from build123d import *

# Parameters (mm, degrees)
F1_DEPTH = 13
F2_W     = 110
F2_H     = 20
F3_DEPTH = 25
F4_W     = 150
F4_H     = 25
F5_DEPTH = 15
F6_R     = 7.5
F7_DEPTH = 25


with BuildPart() as f1:
    # F0 (on Front) → F1 (new body)
    with BuildSketch(Plane.XZ):
        with BuildLine():
            Line((133.362575, 102.236308), (-123.637425, 102.236308))
            ThreePointArc((-123.637425, 102.236308), (-137.779561, 96.378444), (-143.637425, 82.236308))
            Line((-143.637425, 82.236308), (-143.637425, -61.831403))
            Line((-143.637425, -61.831403), (-143.637425, -81.831403))
            Line((-143.637425, -81.831403), (-143.637425, -87.763692))
            ThreePointArc((-143.637425, -87.763692), (-137.779561, -101.905827), (-123.637425, -107.763692))
            Line((-123.637425, -107.763692), (133.362575, -107.763692))
            ThreePointArc((133.362575, -107.763692), (147.50471, -101.905827), (153.362575, -87.763692))
            Line((153.362575, -87.763692), (153.362575, -81.831403))
            Line((153.362575, -81.831403), (153.362575, -61.831403))
            Line((153.362575, -61.831403), (153.362575, 82.236308))
            ThreePointArc((153.362575, 82.236308), (147.50471, 96.378444), (133.362575, 102.236308))
        make_face()
    extrude(amount=F1_DEPTH)

    # F2 (on face) → F3 (cut)
    with BuildSketch(Plane.XZ.offset(13)):
        with Locations((-88.637425, -65.322807)):
            Rectangle(F2_W, F2_H)
        with Locations((98.362575, -65.322807)):
            Rectangle(F2_W, F2_H)
    extrude(amount=-F3_DEPTH, mode=Mode.SUBTRACT)

    # F4 (on face) → F5 (join)
    with BuildSketch(Plane.XZ.offset(13)):
        with Locations((-68.637425, 12.5)):
            Rectangle(F4_W, F4_H)
    extrude(amount=F5_DEPTH)

    # F6 (on face) → F7 (join)
    with BuildSketch(Plane.XZ.offset(13)):
        with Locations((-111.137425, 82.236308)):
            Circle(F6_R)
        with Locations((-91.274098, 82.236308)):
            Circle(F6_R)
        with Locations((-55.741716, 82.236308)):
            Circle(F6_R)
        with Locations((-35.15286, 82.236308)):
            Circle(F6_R)
        with Locations((-4.601658, 82.236308)):
            Circle(F6_R)
        with Locations((22.960842, 82.236308)):
            Circle(F6_R)
    extrude(amount=F7_DEPTH)


solid = f1.part
Could you check a few things on this model? Use its own coordinates, in mm. A direction names the side the tool comes from. Coordinates: 2 decimals unless noted, no trailing zeros. Write each loop counter-clockwise with the first axis right and the second up, starting at its lowest first coordinate (ties: lowest second). Pieces come first, ordered by that corner, then holes. Notation, with made-up numbers: (6, 62) - (47, 62) arc R35 cw to (47, 100) - close; hole circle Ø8 at (-28, 42.25). An arc over 180 degrees is marked (long way). Write item = value, one per line.
1) For faces 1 (the flat face through (43.363, -7, -65)), 2 (the cylindrical face through (-103.984, -25.325, 84.489)), 3 (the flat face through (6.363, -20, 12)), 4 (the flat face through (-33.637, -7, -65)), 5 (the flat face through (-70, -20, 25)), which set-ups out of +Z, -Z, +X, -X, +Y, -Y let a thin tool reach every point of the face, with its end or its side?
Result set:
face_1 = +X, +Y, -Y
face_2 = -Y
face_3 = +Z, -Z, +X, -Y
face_4 = -X, +Y, -Y
face_5 = +X, -X, -Y
2) Please list where these lines run through material, in increasing order: line 1 (Z direction, x = 67, y = -12); line 2 (Y direction, x = 95, z = 18); line 3 (X direction, y = -2.5, z = -68). Write a range as [from, to].
Result set:
line_1 = [-107.76, -75.32], [-55.32, 102.24]
line_2 = [-13, 0]
line_3 = [-33.64, 43.36]
3) Suppose I cut it at B-B on x = -90. Please give me the cut outline in (y, z), plus the area to 3 significant figures.
Result set:
outline = (-38, 74.85) - (-13, 74.85) - (-13, 25) - (-28, 25) - (-28, 0) - (-13, 0) - (-13, -55.32) - (0, -55.32) - (0, 102.24) - (-13, 102.24) - (-13, 89.63) - (-38, 89.63) - close; (-13, -107.76) - (0, -107.76) - (0, -75.32) - (-13, -75.32) - close
area = 3,210 mm2
4) We'd pull the mould along Z, two halves only. Please class faces 6 (the flat face through (-70, -28, 13)), 7 (the flat face through (98, -7, -55.323)), 8 (the flat face through (-89, -7, -75.323)), 9 (the flat face through (-70, -20, 0)): +Z half, -Z half, draft (parallel to the pull), parting line (faces both ways), or undercut.
Result set:
face_6 = draft
face_7 = undercut
face_8 = undercut
face_9 = -Z half
5) Will these pins go through, and if not, where does the flat tip stop? pin 1 Ø7.5 at (x, y) = (-85.5, -23) entering from +Z; pin 2 Ø4 at (x, z) = (45.5, 52.5) entering from -Y; pin 3 Ø7.5 at (x, y) = (-69, -21.5) entering from -Z.
Result set:
pin_1 = 89.46
pin_2 = -13
pin_3 = 0
6) Suppose I cut it at C-C on y = -9.5. Please give me the cut outline in (x, z).
Result set:
outline = (-143.64, -87.76) arc R20 ccw to (-123.64, -107.76) - (133.36, -107.76) arc R20 ccw to (153.36, -87.76) - (153.36, -75.32) - (43.36, -75.32) - (43.36, -55.32) - (153.36, -55.32) - (153.36, 82.24) arc R20 ccw to (133.36, 102.24) - (-123.64, 102.24) arc R20 ccw to (-143.64, 82.24) - (-143.64, -55.32) - (-33.64, -55.32) - (-33.64, -75.32) - (-143.64, -75.32) - close
7) Suppose I cut it at D-D on x = 123. Please give me the cut outline in (y, z).
Result set:
outline = (-13, -107.76) - (0, -107.76) - (0, -75.32) - (-13, -75.32) - close; (-13, -55.32) - (0, -55.32) - (0, 102.24) - (-13, 102.24) - close
8) Suppose I cut it at A-A on y = -23. Please give me the cut outline in (x, z).
Result set:
outline = (-143.64, 0) - (6.36, 0) - (6.36, 25) - (-143.64, 25) - close; circle Ø15 at (-111.14, 82.24); circle Ø15 at (-91.27, 82.24); circle Ø15 at (-55.74, 82.24); circle Ø15 at (-35.15, 82.24); circle Ø15 at (-4.6, 82.24); circle Ø15 at (22.96, 82.24)
